Design review of the part built by this model. Coordinates are the model's own, in mm. A direction names the side the tool comes from. Give positions to 0.01 mm unless a question says otherwise; leave off trailing zeros. Loops run counter-clockwise (first coordinate to the right, second up) from the corner with the lowest first, then second, coordinate; pieces in that order, holes last.
from build123d import *

# Parameters (mm, degrees)
F2_DEPTH       = 500
F1_W           = 38
F1_H           = 13
F3_DEPTH       = 600
F4_T1_DEPTH    = 509.3674969976
F5_R           = 9
F6_R           = 1
F8_DEPTH       = 500.001
F10_DEPTH      = 16.8433111076
F10_DEPTH_BACK = 25


# Not quite as in the source:
# - a fillet or chamfer that OpenCascade refuses, or shapes differently, is made with other operations: its cross-section is extruded or revolved along the edge and cut away or added
# - ends of sketch curves that miss each other by under 0.0002 mm in the source are joined


with BuildPart() as f2:
    # F0 (on Front) → F2 (new body)
    with BuildSketch(Plane.XZ):
        with BuildLine():
            Line((22.5, 5.3759940737), (0, 5.3759940737))
            Line((0, 5.3759940737), (-22.5, 5.3759940737))
            Line((-22.5, 5.3759940737), (-22.5, 6.6759940737))
            Line((-22.5, 6.6759940737), (-45.5824640741, 6.6759940737))
            Line((-45.5824640741, 6.6759940737), (-57.5, -3.3240059263))
            Line((-57.5, -3.3240059263), (-57.5, -7.3240059263))
            Line((-57.5, -7.3240059263), (-40.1794919243, -17.3240059263))
            ThreePointArc((-40.1794919243, -17.3240059263), (0, -13.2464610679), (40.1794919243, -17.3240059263))
            Line((40.1794919243, -17.3240059263), (57.5, -7.3240059263))
            Line((57.5, -7.3240059263), (57.5, -3.3240059263))
            Line((57.5, -3.3240059263), (45.5824640741, 6.6759940737))
            Line((45.5824640741, 6.6759940737), (22.5, 6.6759940737))
            Line((22.5, 6.6759940737), (22.5, 5.3759940737))
        make_face()
    extrude(amount=F2_DEPTH)

    # F1 (on face) → F3 (cut)
    with BuildSketch(Plane.XZ):
        with Locations((0, -3.1240059263)):
            Rectangle(F1_W, F1_H)
    extrude(amount=F3_DEPTH, mode=Mode.SUBTRACT)

    # F4: fillet of radius 2 on 2 edges, made by hand

    # F4_s2 → F4_t1 (cut)
    with BuildSketch(Plane.XZ.offset(-4.6837484988)):
        with BuildLine():
            ThreePointArc((-24.3734993995, 6.6759940737), (-23.2333239744, 6.3191617462), (-22.5, 5.3759940737))
            Line((-22.5, 5.3759940737), (-22.5, 6.6759940737))
            Line((-22.5, 6.6759940737), (-24.3734993995, 6.6759940737))
        make_face()
        with BuildLine():
            ThreePointArc((24.3734993995, 6.6759940737), (23.2333239744, 6.3191617462), (22.5, 5.3759940737))
            Line((22.5, 5.3759940737), (22.5, 6.6759940737))
            Line((22.5, 6.6759940737), (24.3734993995, 6.6759940737))
        make_face()
    extrude(amount=F4_T1_DEPTH, mode=Mode.SUBTRACT)

    # F5
    f5_edges = [f2.edges().sort_by_distance(p)[0] for p in [
        (-45.582464, -250, 6.675994),
        (-40.179492, -250, -17.324006),
        (40.179492, -250, -17.324006),
        (45.582464, -250, 6.675994),
    ]]
    fillet(f5_edges, radius=F5_R)

    # F6
    f6_edges = [f2.edges().sort_by_distance(p)[0] for p in [
        (57.5, -250, -3.324006),
        (57.5, -250, -7.324006),
        (-57.5, -250, -7.324006),
        (-57.5, -250, -3.324006),
    ]]
    fillet(f6_edges, radius=F6_R)

    # F7 (on face) → F8 (cut, through all)
    with BuildSketch(Plane.XZ.offset(500)):
        with BuildLine():
            ThreePointArc((-42.1022688854, -13.9044885758), (-39.7790672738, -14.7426835793), (-37.3093702039, -14.7218755322))
            ThreePointArc((-37.3093702039, -14.7218755322), (-29.1789784784, -13.3650277579), (-20.9999997169, -12.3410102235))
            Line((-20.9999997169, -12.3410102235), (-20.9999997169, 3.3759940737))
            Line((-20.9999997169, 3.3759940737), (-22.5, 3.3759940737))
            ThreePointArc((-22.5, 3.3759940737), (-23.2333240923, 4.3191614627), (-24.3734993995, 4.67599366))
            Line((-24.3734993995, 4.67599366), (-42.3067319657, 4.67599366))
            ThreePointArc((-42.3067319657, 4.67599366), (-44.7008728275, 4.2538420304), (-46.8062449676, 3.0383048586))
            Line((-46.8062449676, 3.0383048586), (-55.4999995863, -4.2566214356))
            Line((-55.4999995863, -4.2566214356), (-55.4999995863, -6.1693051491))
            Line((-55.4999995863, -6.1693051491), (-42.1022688854, -13.9044885758))
        make_face()
        with BuildLine():
            Line((20.9999997169, 3.3759940737), (20.9999997169, -12.3410102235))
            ThreePointArc((20.9999997169, -12.3410102235), (29.1789784784, -13.3650277579), (37.3093702039, -14.7218755322))
            ThreePointArc((37.3093702039, -14.7218755322), (39.7790673581, -14.7426840737), (42.1022691362, -13.9044890102))
            Line((42.1022691362, -13.9044890102), (55.5000000879, -6.1693054387))
            Line((55.5000000879, -6.1693054387), (55.5000000879, -4.2566212017))
            Line((55.5000000879, -4.2566212017), (46.8062452899, 3.0383052428))
            ThreePointArc((46.8062452899, 3.0383052428), (44.700872999, 4.2538425017), (42.3067319657, 4.6759941615))
            Line((42.3067319657, 4.6759941615), (24.3734993995, 4.6759941615))
            ThreePointArc((24.3734993995, 4.6759941615), (23.2333239494, 4.3191618064), (22.5, 3.3759940737))
            Line((22.5, 3.3759940737), (20.9999997169, 3.3759940737))
        make_face()
    extrude(amount=-F8_DEPTH, mode=Mode.SUBTRACT)

    # F9 (on Top) → F10 (cut, two sides)
    with BuildSketch(Plane.XY) as f10_sk:
        with BuildLine():
            ThreePointArc((-57.495400138, -49.2727015938), (0.3636564761, 7.498850023), (57.5, -50))
            Line((57.5, -50), (57.8162293472, 0))
            Line((57.8162293472, 0), (57.8162293472, 30))
            Line((57.8162293472, 30), (-57.1837706528, 30))
            Line((-57.1837706528, 30), (-57.1837706528, 0))
            Line((-57.1837706528, 0), (-57.495400138, -49.2727015938))
        make_face()
    extrude(amount=-F10_DEPTH, mode=Mode.SUBTRACT)
    extrude(f10_sk.sketch, amount=F10_DEPTH_BACK, mode=Mode.SUBTRACT)


solid = f2.part
Q1. Take a section at B-B (y = -199.5). Give the number of separate pieces and of enclosed holes in the cut face, plus the area to 3 significant figures.
Results:
separate pieces: 1
enclosed holes: 3
area: 622 mm2
Q2. Tool access review of faces 4 (the face through (-33, -254, 4.676)), 5 (the face through (0, -500, -10)): name each direction out of +Z, -Z, +X, -X, +Y, -Y from which nothing blocks a thin tool from reaching the whole face with its end or side.
Results:
face 4: +Y, -Y
face 5: +Z, -Z, +X, -X, -Y
Q3. Take a section at A-A (x = -12.5). Give the boundary of the cut face in (y, z).
Results:
outline: (-500, -13.64) - (0, -13.64) - (0, -9.62) - (-500, -9.62) - close; (-500, 3.38) - (0, 3.38) - (0, 5.38) - (-500, 5.38) - close
Q4. Draft analysis for pull direction Z (two halves, no side actions). For faces 1 (the face through (51.214, -261.685, -0.66)), 2 (the face through (0, 0, -12)), 3 (the face through (-52.55, -255.87, 0.83)), state which applies: pulls with the +Z half, pulls with the -Z half, needs draft (parallel to the pull), parting line crosses it, or undercut.
Results:
face 1: undercut
face 2: needs draft
face 3: pulls with the +Z half
Q5. Insertion check: pin 1 (1.5 mm diameter, centred on y = -265.5, z = -12, fed in from +X); pin 2 (8 mm diameter, centred on y = -109, z = 2.5, fed in from +X); pin 3 (1.7 mm diameter, centred on x = -21.5, y = -204, fed in from -Z). Each pin has a flat end and moves straight along its axis. Give the tip position at first contact, or say it passes through.
Results:
pin 1: stops at x = 50.7
pin 2: stops at x = 55.33
pin 3: stops at z = -14.5
Q6. Wall thickness on line 1 (X direction, y = -424, z = -5.25); line 2 (Z direction, x = -0.5, y = -186.5); line 3 (X direction, y = -278.5, z = 0.75): over which ranges is each line inside the solid? List them lowest first.
Results:
line 1: x = -57.5 to -55.5, -21 to -19, 19 to 21, 55.5 to 57.5
line 2: z = -13.25 to -9.62, 3.38 to 5.38
line 3: x = -52.64 to -49.53, -21 to -19, 19 to 21, 49.53 to 52.64
